Check sheet for the drawn part. Datum: minimum x, y, z corner. Units: mm. Round coordinates to 2 decimals unless told otherwise and drop trailing zeros. Order: outer loops, then holes, each group sorted by start corner. A loop starts at its lowest first (then second) coordinate and runs counter-clockwise, first axis right, second up. Notation, with made-up numbers: M 72,70.25 L 83,70.25 A25 ccw 83,82.25 Z; hole C 7.5,77.5 d3. An arc over 180 degrees is marked long. Write item = value, one per line. Start each with the question number.
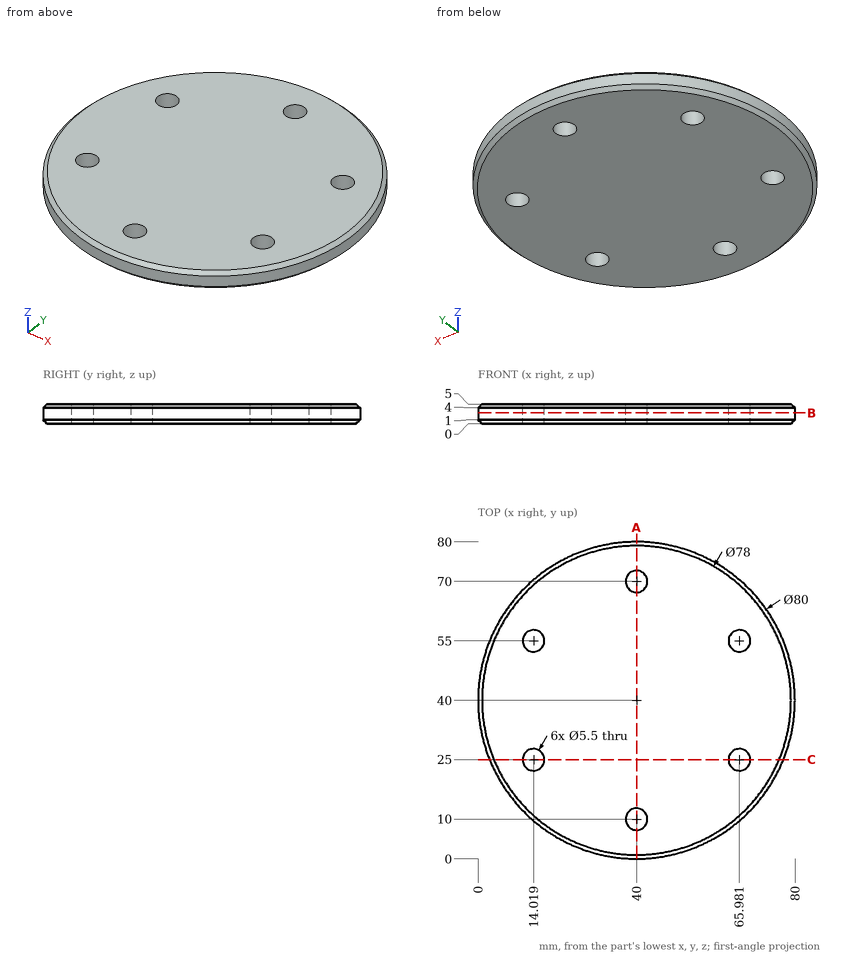
1) Cross-section at C-C, the plane y = 25. Give the number of separate pieces and of enclosed holes in the cut face, then the cut area to 3 significant figures.
2) Cross-section at A-A, the plane x = 40. Enter the section's corners in (y, z).
3) Cross-section at B-B, the plane z = 2.75. Enter the section's corners in (x, y).
4) Gauge pin test, flat ends, axial feed: P1, Ø5, axis at x = 14.02, y = 55, coming from the +Z side; P2, Ø3, axis at x = 54.5, z = 1, coming from the +Y side; P3, Ø2, axis at y = 38, z = 2.5, coming from the +X side. Record the tip position at first contact, or that the pin passes through.
5) Scan lines: probe 1 along X at (y, z) = (55, 1); probe 2 along X at (y, z) = (26.5, 3.85) (1 decimal); probe 3 along Y at (x, z) = (41, 0.9). Record each from-to range of solid material in increasing order.
Geometry results:
q1.separate_pieces = 3
q1.enclosed_holes = 0
q1.area = 314 mm^2
q2.outline = M 0,1 L 1,0 L 7.25,0 L 7.25,5 L 1,5 L 0,4 Z; M 12.75,0 L 67.25,0 L 67.25,5 L 12.75,5 Z; M 72.75,0 L 79,0 L 80,1 L 80,4 L 79,5 L 72.75,5 Z
q3.outline = C 40,40 d80; hole C 14.02,25 d5.5; hole C 14.02,55 d5.5; hole C 40,10 d5.5; hole C 40,70 d5.5; hole C 65.98,25 d5.5; hole C 65.98,55 d5.5
q4.P1 = through
q4.P2 = 77.83
q4.P3 = 79.99
q5.probe_1 = 2.92 to 11.27, 16.77 to 63.23, 68.73 to 77.08
q5.probe_2 = 2.3 to 11.7, 16.3 to 63.7, 68.3 to 77.7
q5.probe_3 = 0.11 to 7.44, 12.56 to 67.44, 72.56 to 79.89
